Verification items for this drawing (mm, ordinates from the low corner). A direction names the side the tool comes from. Coordinates: 2 decimals unless noted, no trailing zeros. Loops run counter-clockwise (first coordinate to the right, second up) from the corner with the lowest first, then second, coordinate; pieces in that order, holes last. Notation, with made-up numbers: (18, 56) - (64, 56) arc R18 cw to (64, 81) - close; hole circle Ø7 at (-2.75, 63). An arc over 180 degrees is marked (long way). Write each question's results on one line, items separated by ' | '. Start each with the question number.
(1) Access from +Z, -Z, +X, -X, +Y, -Y to the whole of each face (thin tool, end or side, straight path). Record for the marked faces 1 and 2.
(2) Sectioned sample at A-A (y = 10.25). Enter the section's corners in (x, z), plus the area to 3 significant figures.
(3) Mould release check, pull along X, two halves, no side actions. Record for the marked faces 3, 4 and 5: pulls with the +X half, pulls with the -X half, needs draft (parallel to the pull), parting line crosses it, or undercut.
(4) Material ranges on probe 1 along Z at (x, y) = (85.5, 11.5); probe 2 along X at (y, z) = (3.5, 9); probe 3 along Y at (x, z) = (75, 64), recorded low to high.
(5) Go/stop test with a flat-tipped pin: pin 1 Ø3 at (x, z) = (33, 98.5) entering from -Y. Record where the tip stops, or that it passes through.
(6) Sectioned sample at C-C (z = 67). Enter the section's corners in (x, y), plus the area to 3 significant figures.
(7) Sectioned sample at B-B (x = 71). Enter the section's corners in (y, z), plus the area to 3 significant figures.
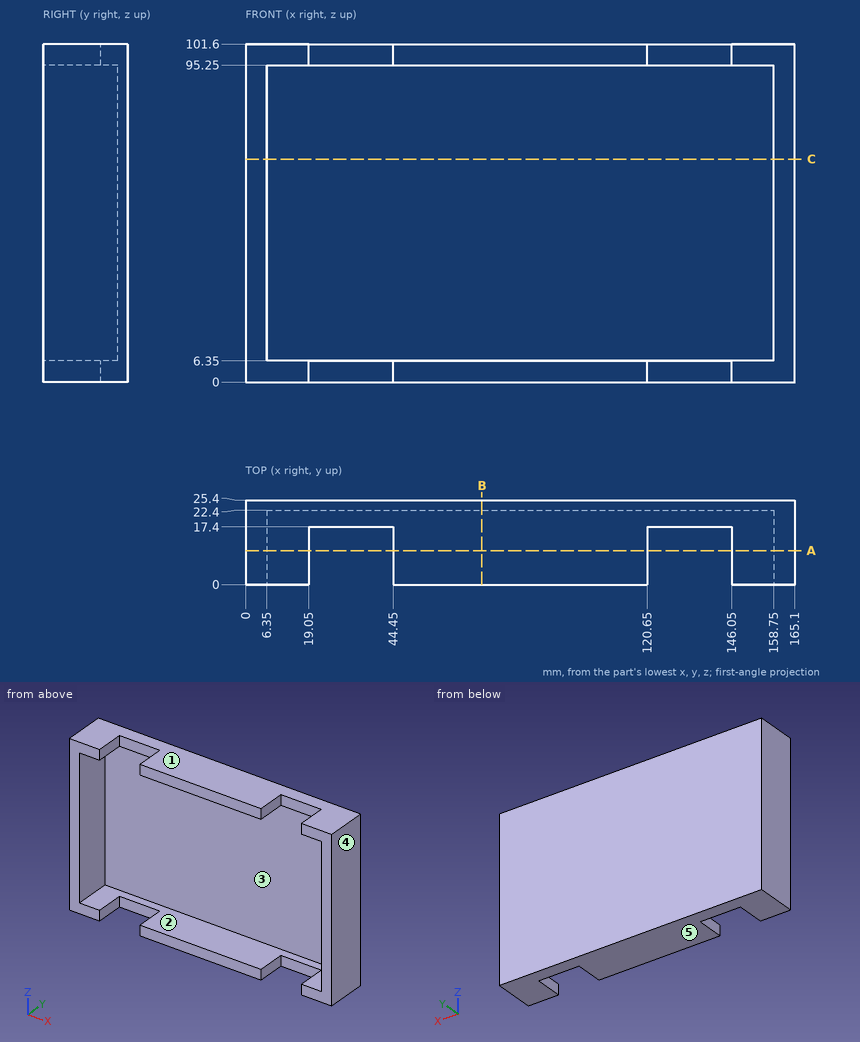
Outcome:
1) face 1: +Z, +X, -X, +Y, -Y | face 2: -Y
2) outline: (0, 0) - (19.05, 0) - (19.05, 6.35) - (6.35, 6.35) - (6.35, 95.25) - (19.05, 95.25) - (19.05, 101.6) - (0, 101.6) - close; (44.45, 0) - (120.65, 0) - (120.65, 6.35) - (44.45, 6.35) - close; (44.45, 95.25) - (120.65, 95.25) - (120.65, 101.6) - (44.45, 101.6) - close; (146.05, 0) - (165.1, 0) - (165.1, 101.6) - (146.05, 101.6) - (146.05, 95.25) - (158.75, 95.25) - (158.75, 6.35) - (146.05, 6.35) - close | area: 2,580 mm2
3) face 3: undercut | face 4: pulls with the +X half | face 5: needs draft
4) probe 1: z = 0 to 6.35, 95.25 to 101.6 | probe 2: x = 0 to 6.35, 158.75 to 165.1 | probe 3: y = 22.4 to 25.4
5) pin 1: stops at y = 17.4
6) outline: (0, 0) - (6.35, 0) - (6.35, 22.4) - (158.75, 22.4) - (158.75, 0) - (165.1, 0) - (165.1, 25.4) - (0, 25.4) - close | area: 780 mm2
7) outline: (0, 0) - (25.4, 0) - (25.4, 101.6) - (0, 101.6) - (0, 95.25) - (22.4, 95.25) - (22.4, 6.35) - (0, 6.35) - close | area: 589 mm2
